The model under review builds one solid part; all positions refer to its coordinate system, in mm. Face numbers are marked on the shaded views. A direction names the side the tool comes from. Coordinates: 2 decimals unless noted, no trailing zeros. Write each loop counter-clockwise with the first axis right and the second up, starting at its lowest first coordinate (ties: lowest second). Pieces come first, ordered by that corner, then holes. Notation, with made-up numbers: M 47,59 L 61,59 A23 ccw 61,91 Z; hole C 79.25,-21.75 d6. An arc over 180 degrees is marked long. Answer as a JSON object with one key per item and string values.
```python
from build123d import *

# Parameters (mm, degrees)
CROQUIS1_W              = 200
CROQUIS1_H              = 170
SALIENTE_EXTRUIR1_DEPTH = 10
CROQUIS2_W              = 59.79
CROQUIS2_H              = 10
CROQUIS2_W_2            = 30.21
SALIENTE_EXTRUIR2_DEPTH = 150
CROQUIS3_W              = 90
CROQUIS3_H              = 10
SALIENTE_EXTRUIR3_DEPTH = 100
CROQUIS4_W              = 5.25
CROQUIS4_H              = 5.5
CORTAR_EXTRUIR1_DEPTH   = 170
CROQUIS7_W              = 90
CROQUIS7_H              = 10
SALIENTE_EXTRUIR4_DEPTH = 5
CORTAR_EXTRUIR3_DEPTH   = 10
CORTAR_EXTRUIR4_DEPTH   = 30
CORTAR_EXTRUIR5_DEPTH   = 5
CROQUIS10_W             = 30
CROQUIS10_H             = 13.5
CROQUIS10_W_2           = 24
CROQUIS10_H_2           = 8
SALIENTE_EXTRUIR5_DEPTH = 4.3
CROQUIS11_R             = 1.1
CORTAR_EXTRUIR6_DEPTH   = 14.3
CROQUIS12_R             = 1.75
CORTAR_EXTRUIR7_DEPTH   = 6.4
CROQUIS13_R             = 1.7
CORTAR_EXTRUIR8_DEPTH   = 5
CROQUIS14_W             = 0.3
CROQUIS14_H             = 10
CORTAR_EXTRUIR9_DEPTH   = 5
SALIENTE_EXTRUIR6_DEPTH = 5


with BuildPart() as part:
    # Croquis1 → Saliente-Extruir1 (new body)
    with BuildSketch(Plane(origin=(0, 0, 0), x_dir=(1, 0, 0), z_dir=(0, 1, 0))):
        Rectangle(CROQUIS1_W, CROQUIS1_H)
    extrude(amount=SALIENTE_EXTRUIR1_DEPTH)

    # Croquis2 → Saliente-Extruir2 (add)
    with BuildSketch(Plane(origin=(0, 10, 0), x_dir=(1, 0, 0), z_dir=(0, 1, 0))):
        Polygon((-100, 85), (-100, -85), (-90, -85), (-90, -75), (-90, 75), (-90, 85), align=None)
        Polygon((100, 85), (90, 85), (90, 75), (90, -75), (90, -85), (100, -85), align=None)
        with Locations((-60.105, -80)):
            Rectangle(CROQUIS2_W, CROQUIS2_H)
        with Locations((74.895, -80)):
            Rectangle(CROQUIS2_W_2, CROQUIS2_H)
    extrude(amount=SALIENTE_EXTRUIR2_DEPTH)

    # Croquis3 → Saliente-Extruir3 (add)
    with BuildSketch(Plane(origin=(0, 160, 0), x_dir=(1, 0, 0), z_dir=(0, 1, 0))):
        with Locations((14.79, -80)):
            Rectangle(CROQUIS3_W, CROQUIS3_H)
    extrude(amount=-SALIENTE_EXTRUIR3_DEPTH)

    # Croquis4 → Cortar-Extruir1 (cut)
    with BuildSketch(Plane(origin=(0, 10, 65), x_dir=(-1, 0, 0), z_dir=(0, 1, 0))):
        with Locations((92.625, -145)):
            Rectangle(CROQUIS4_W, CROQUIS4_H)
        with Locations((-92.625, -145)):
            Rectangle(CROQUIS4_W, CROQUIS4_H)
    extrude(amount=CORTAR_EXTRUIR1_DEPTH, mode=Mode.SUBTRACT)

    # Croquis7 → Saliente-Extruir4 (add)
    with BuildSketch(Plane.XY.offset(85)):
        with Locations((14.79, 65)):
            Rectangle(CROQUIS7_W, CROQUIS7_H)
    extrude(amount=SALIENTE_EXTRUIR4_DEPTH)

    # Croquis8 → Cortar-Extruir3 (cut)
    with BuildSketch(Plane(origin=(0, 160, 0), x_dir=(1, 0, 0), z_dir=(0, 1, 0))):
        Polygon((98, 70), (98, -83), (-98, -83), (-98, 70), (-92, 70), (-92, -77), (92, -77), (92, 70), align=None)
    extrude(amount=-CORTAR_EXTRUIR3_DEPTH, mode=Mode.SUBTRACT)

    # Croquis9 → Cortar-Extruir4 (cut)
    with BuildSketch(Plane(origin=(0, 10, 0), x_dir=(1, 0, 0), z_dir=(0, 1, 0))):
        Polygon((-95.25, 77.25), (-95.25, 82.75), (-71.25, 82.75), (-71.25, 77.25), (-71.25, 74.75), (-95.25, 74.75), align=None)
    extrude(amount=-CORTAR_EXTRUIR4_DEPTH, mode=Mode.SUBTRACT)

    # Croquis9_2 → Cortar-Extruir5 (cut)
    with BuildSketch(Plane(origin=(0, 10, 0), x_dir=(1, 0, 0), z_dir=(0, 1, 0))):
        Polygon((-95.25, 77.25), (-95.25, 82.75), (-71.25, 82.75), (-71.25, 77.25), (-71.25, 74.75), (-95.25, 74.75), align=None)
    extrude(amount=CORTAR_EXTRUIR5_DEPTH, mode=Mode.SUBTRACT)

    # Croquis10 → Saliente-Extruir5 (add)
    with BuildSketch(Plane.XZ):
        with Locations((-83.25, -78.5)):
            Rectangle(CROQUIS10_W, CROQUIS10_H)
        with Locations((-83.25, -78.75)):
            Rectangle(CROQUIS10_W_2, CROQUIS10_H_2, mode=Mode.SUBTRACT)
    extrude(amount=SALIENTE_EXTRUIR5_DEPTH)

    # Croquis11 → Cortar-Extruir6 (cut)
    with BuildSketch(Plane.XY.offset(-71.75)):
        with Locations((-77.55, -2.1)):
            Circle(CROQUIS11_R)
        with Locations((-86.93, -2.1)):
            Circle(CROQUIS11_R)
    extrude(amount=-CORTAR_EXTRUIR6_DEPTH, mode=Mode.SUBTRACT)

    # Croquis12 → Cortar-Extruir7 (cut)
    with BuildSketch(Plane.XZ):
        with Locations((-91.5, -55)):
            Circle(CROQUIS12_R)
        with Locations((18.5, -55)):
            Circle(CROQUIS12_R)
        with Locations((-91.5, 55)):
            Circle(CROQUIS12_R)
        with Locations((18.5, 55)):
            Circle(CROQUIS12_R)
    extrude(amount=-CORTAR_EXTRUIR7_DEPTH, mode=Mode.SUBTRACT)

    # Croquis13 → Cortar-Extruir8 (cut)
    with BuildSketch(Plane.XY.offset(85)):
        with Locations((-50.21, 24)):
            Circle(CROQUIS13_R)
        with Locations((79.79, 24)):
            Circle(CROQUIS13_R)
    extrude(amount=-CORTAR_EXTRUIR8_DEPTH, mode=Mode.SUBTRACT)

    # Croquis14 → Cortar-Extruir9 (cut)
    with BuildSketch(Plane.XY.offset(90)):
        with Locations((-30.06, 65)):
            Rectangle(CROQUIS14_W, CROQUIS14_H)
        with Locations((59.64, 65)):
            Rectangle(CROQUIS14_W, CROQUIS14_H)
    extrude(amount=-CORTAR_EXTRUIR9_DEPTH, mode=Mode.SUBTRACT)

    # Croquis15 → Saliente-Extruir6 (add)
    with BuildSketch(Plane.XY.offset(85)):
        Polygon((14.79, 0), (94.79, 0), (94.79, 4.8), (14.79, 4.8), (-65.21, 4.8), (-65.21, 0), align=None)
    extrude(amount=SALIENTE_EXTRUIR6_DEPTH)


solid = part.part
```
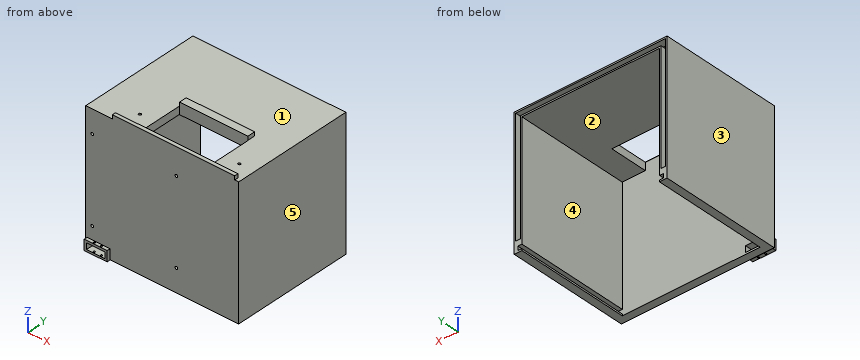
(1) For pin 1 Ø1 at (x, z) = (-29, 26) entering from +Y; pin 2 Ø5 at (x, z) = (2.5, 6.5) entering from -Y; pin 3 Ø2.5 at (x, y) = (-50.5, 24) entering from +Z, all flat-tipped, find the tip position at first contact; note any pin that passes through.
Results list:
{"pin 1": "y = 10", "pin 2": "y = 0", "pin 3": "z = 80"}
(2) For the marked faces 4 and 5, list the 3-axis set-ups (+Z, -Z, +X, -X, +Y, -Y) from which the entire face can be reached by the end or side of a thin tool; tool diameter is ignored.
Results list:
{"face 4": "-Z, +Y", "face 5": "+Z, -Z, +X, +Y, -Y"}
(3) Draft analysis for pull direction X (two halves, no side actions). For the marked faces 1, 2 and 3, state which applies: released by +X, released by -X, zero draft, split by the parting line, or undercut.
Results list:
{"face 1": "zero draft", "face 2": "undercut", "face 3": "released by -X"}
(4) Add section A-A on x = 36.5. Give the boundary of the cut face in (y, z), and give its area (3 significant figures).
Results list:
{"outline": "M 0,-85 L 10,-85 L 10,85 L 4.8,85 L 4.8,90 L 0,90 Z; M 60,75 L 160,75 L 160,77 L 150,77 L 150,83 L 160,83 L 160,85 L 70,85 L 70,90 L 60,90 Z", "area": "2,710 mm²"}
(5) Wall thickness on line 1 along Z through (x, y) = (-91.5, 2); line 2 along Z through (x, y) = (18.5, 5); line 3 along Z through (x, y) = (18.5, 1.5): over which ranges is each line inside the solid? List them lowest first. Write a range as from..to.
Results list:
{"line 1": "-85..-82.75, -74.75..-56.75, -53.25..53.25, 56.75..85", "line 2": "-85..-56.75, -53.25..53.25, 56.75..85", "line 3": "-85..-56.75, -53.25..53.25, 56.75..90"}
(6) Add section C-C on z = 68. Give the boundary of the cut face in (x, y), and give its area (3 significant figures).
Results list:
{"outline": "M -100,0 L 100,0 L 100,160 L 98,160 L 98,150 L 92,150 L 92,160 L 90,160 L 90,10 L -90,10 L -90,160 L -92,160 L -92,150 L -98,150 L -98,160 L -100,160 Z", "area": "4,880 mm²"}
(7) Add section D-D on x = -57. Give the boundary of the cut face in (y, z), and give its area (3 significant figures).
Results list:
{"outline": "M 0,-85 L 10,-85 L 10,75 L 160,75 L 160,77 L 150,77 L 150,83 L 160,83 L 160,85 L 4.8,85 L 4.8,90 L 0,90 Z", "area": "3,160 mm²"}
(8) Add section B-B on y = 75.5. Give the boundary of the cut face in (x, z).
Results list:
{"outline": "M -100,-85 L -90,-85 L -90,-82.75 L -95.25,-82.75 L -95.25,-77.25 L -90,-77.25 L -90,75 L 90,75 L 90,-77.25 L 95.25,-77.25 L 95.25,-82.75 L 90,-82.75 L 90,-85 L 100,-85 L 100,85 L -100,85 Z"}
